Work out the finished part from the listing and answer in its coordinate system (mm). Face numbers are marked on the shaded views. A direction names the side the tool comes from. Coordinates: 2 decimals unless noted, no trailing zeros. Loops run counter-clockwise (first coordinate to the right, second up) from the corner with the lowest first, then second, coordinate; pieces in that order, holes last.
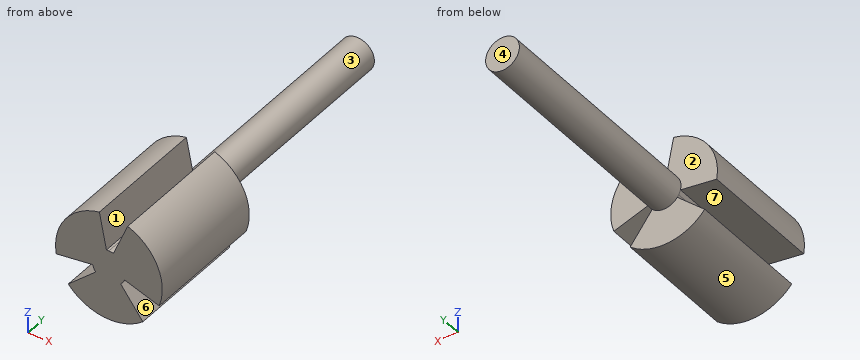
```python
from build123d import *

# Parameters (mm, degrees)
SKETCH1_R           = 9.5
BOSS_EXTRUDE1_DEPTH = 200
SKETCH2_R           = 30
SKETCH2_R_2         = 9.5
BOSS_EXTRUDE2_DEPTH = 70
CUT_EXTRUDE1_DEPTH  = 137.747943312
CIRPATTERN1_COUNT   = 3


with BuildPart() as part:
    # Sketch1 → Boss-Extrude1 (new body)
    with BuildSketch(Plane(origin=(0, 0, 0), x_dir=(1, 0, 0), z_dir=(0, 1, 0))):
        with Locations(Location((0, 0, 0), (0, 0, 270))):
            Circle(SKETCH1_R)
    extrude(amount=BOSS_EXTRUDE1_DEPTH)

    # Sketch2 → Boss-Extrude2 (add)
    with BuildSketch(Plane.XZ):
        with Locations(Location((0, 0, 0), (0, 0, 270))):
            Circle(SKETCH2_R)
        with Locations(Location((0, 0, 0), (0, 0, 270))):
            Circle(SKETCH2_R_2, mode=Mode.SUBTRACT)
    extrude(amount=-BOSS_EXTRUDE2_DEPTH)

    # Sketch3 → Cut-Extrude1 (cut, through all)
    with BuildSketch(Plane(origin=(0, 70, 0), x_dir=(1, 0, 0), z_dir=(0, 1, 0))):
        Polygon((-5.921460856, -32.258084995), (-1.382914739, -9.398805606), (0, -9.5), (2.553944051, -9.150266104), (12.286259273, -32.258084995), align=None)
    cut_extrude1 = extrude(amount=-CUT_EXTRUDE1_DEPTH, mode=Mode.SUBTRACT)

    # CirPattern1: Cut-Extrude1 ×3 about axis
    cirpattern1_axis = Axis((0, 0, 0), (0, 1, 0))
    for i in range(1, CIRPATTERN1_COUNT):
        add(cut_extrude1.rotate(cirpattern1_axis, i * 360 / CIRPATTERN1_COUNT), mode=Mode.SUBTRACT)


solid = part.part
```
1. Each of these flat-tipped pins is pushed along its axis until it touches: P1, Ø3, axis at y = 156, z = 11.5, coming from the +X side; P2, Ø2, axis at y = 48.5, z = 5.5, coming from the +X side; P3, Ø22, axis at x = 20.5, z = 14, coming from the +Y side; P4, Ø1, axis at y = 136, z = -1.5, coming from the +X side. Where does it stop, or does it pass through?
2. A cutting plane is placed at D-D, the plane x = 25.5. Give the vertices of the cut face in (y, z).
3. A cutting plane is placed at C-C, the plane z = 0. Give the vertices of the cut face in (x, y).
4. Straight lines are drawn through the part: probe 1 along Y at (x, z) = (-8, 16); probe 2 along Z at (x, y) = (-2.5, 83); probe 3 along Z at (x, y) = (7, 12.5). For each, find the intervals that lie inside material, in ascending order.
5. A cutting plane is placed at B-B, the plane z = 24. Give the vertices of the cut face in (x, y), then the cut area to 3 significant figures.
6. For the marked faces 1, 2 and 3, determine the directions among +Z, -Z, +X, -X, +Y, -Y from which every point of the face is accessible in a straight line to the end or side of a thin tool.
7. Determine the mould class of the marked faces 4, 5, 6 and 7 for opening direction X: released by +X, released by -X, zero draft, split by the parting line, or undercut.
8. A cutting plane is placed at A-A, the plane y = 33. Give the vertices of the cut face in (x, z).
Answers below:
1. P1: passes through
1. P2: stops at x = 29.66
1. P3: stops at y = 70
1. P4: stops at x = 9.45
2. outline: (0, -9.17) - (70, -9.17) - (70, 15.8) - (0, 15.8) - close
3. outline: (-30, 0) - (30, 0) - (30, 70) - (9.5, 70) - (9.5, 200) - (-9.5, 200) - (-9.5, 70) - (-30, 70) - close
4. probe 1: y = 0 to 70
4. probe 2: z = -9.17 to 9.17
4. probe 3: z = -29.17 to -7.25, -6.33 to 19.71
5. outline: (-18, 0) - (-4.28, 0) - (-4.28, 70) - (-18, 70) - close; (8.81, 0) - (18, 0) - (18, 70) - (8.81, 70) - close
5. area: 1,600 mm2
6. face 1: +Z, +Y, -Y
6. face 2: +Z, -X, +Y
6. face 3: +Y
7. face 4: zero draft
7. face 5: split by the parting line
7. face 6: undercut
7. face 7: undercut
8. outline: (-29.59, -4.93) - (-9.2, -2.36) - (-8.23, -4.75) - (-7.45, -5.9) - (-22.87, -19.41) arc R30 ccw to (19.06, -23.17) - (6.65, -6.79) - (8.23, -4.75) - (8.83, -3.5) - (28.25, -10.1) arc R30 ccw to (10.53, 28.09) - (2.55, 9.15) - (0, 9.5) - (-1.38, 9.4) - (-5.38, 29.51) arc R30 ccw to start
